Read the model definition and answer for the solid it produces. Units are mm, in the model's axes. Face numbers are marked on the shaded views. Round coordinates to 2 decimals unless told otherwise and drop trailing zeros. Order: outer loops, then holes, each group sorted by start corner. A loop starts at its lowest first (then second) coordinate and runs counter-clockwise, first axis right, second up. Notation, with made-up numbers: (46, 37) - (82, 37) arc R10 cw to (82, 44) - close; hole circle Ø2 at (32, 85.25). An arc over 180 degrees is marked (long way). Answer as a JSON object with one key per item and string values. Group by question number.
Q1. A cutting plane is placed at A-A on y = -93.5. Determine the outline of the cut face in (x, z), and give its area (3 significant figures).
Q2. A cutting plane is placed at C-C on x = -16. Determine the outline of the cut face in (y, z).
Q3. A cutting plane is placed at B-B on z = 5.5. Determine the outline of the cut face in (x, y).
Q4. Consider line 1 (Y direction, x = -47.5, z = 4.25); line 2 (X direction, y = -6, z = 6); line 3 (Z direction, x = -73, y = 64). Determine where each line is inside the solid, lowest interval first.
Q5. Given pin 1 Ø12 at (x, y) = (107, 92) entering from -Z; pin 2 Ø2.5 at (x, y) = (-133.08, 91.92) entering from -Z; pin 3 Ø10 at (x, y) = (70.5, 71.5) entering from +Z, each flat-ended and moving along its own axis, determine where each tip first touches the part or whether it passes through.
Q6. The mould has two halves that part along Y. Classify the marked faces 1 and 2: pulls with the +Y half, pulls with the -Y half, needs draft (parallel to the pull), parting line crosses it, or undercut.
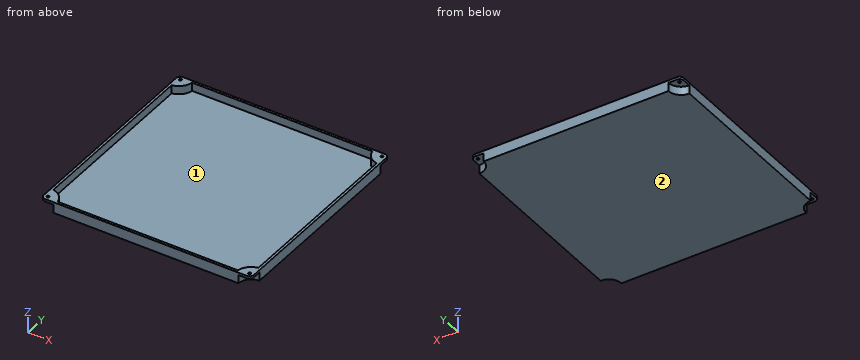
Autodesk Inventor part; units mm, degrees
ref_plane "YZ Plane" through (0, 0, 0) normal (1, 0, 0) x (0, 1, 0)
ref_plane "XZ Plane" through (0, 0, 0) normal (0, 1, 0) x (-1, 0, 0)
ref_plane "XY Plane" through (0, 0, 0) normal (0, 0, 1) x (1, 0, 0)
sketch "Sketch1" plane through (0, 0, 0) normal (0, 0, 1) x (1, 0, 0)
  line L0 (-123.0769, 96.9231) -> (96.9231, 96.9231)
  line L1 (111.9231, 81.9231) -> (111.9231, -138.0769)
  line L2 (96.9231, -153.0769) -> (-123.0769, -153.0769)
  line L3 (-138.0769, -138.0769) -> (-138.0769, 81.9231)
  arc A0 (-138.0769, 81.9231) -> (-123.0769, 96.9231) centre (-138.0769, 96.9231) ccw
  arc A1 (96.9231, 96.9231) -> (111.9231, 81.9231) centre (111.9231, 96.9231) ccw
  arc A2 (111.9231, -138.0769) -> (96.9231, -153.0769) centre (111.9231, -153.0769) ccw
  arc A3 (-123.0769, -153.0769) -> (-138.0769, -138.0769) centre (-138.0769, -153.0769) ccw
  point P0 (0, 0)
  dimension "d4" = 30
  dimension "d5" = 30
  dimension "d6" = 30
  dimension "d7" = 30
  dimension "d27" = 250
  dimension "d28" = 250
extrude "Extrusion1" add sketch "Sketch1" along normal blind 3
sketch "Sketch2" plane through (0, 0, 3) normal (0, 0, 1) x (1, 0, 0)
  line L0 (-123.0769, -153.0769) -> (96.9231, -153.0769)
  arc A0 (111.9231, -138.0769) -> (96.9231, -153.0769) centre (111.9231, -153.0769) ccw
  line L1 (111.9231, -138.0769) -> (111.9231, 81.9231)
  arc A1 (96.9231, 96.9231) -> (111.9231, 81.9231) centre (111.9231, 96.9231) ccw
  line L2 (96.9231, 96.9231) -> (-123.0769, 96.9231)
  arc A2 (-138.0769, 81.9231) -> (-123.0769, 96.9231) centre (-138.0769, 96.9231) ccw
  line L3 (-138.0769, 81.9231) -> (-138.0769, -138.0769)
  arc A3 (-123.0769, -153.0769) -> (-138.0769, -138.0769) centre (-138.0769, -153.0769) ccw
  line L4 (-120.3287, 93.9231) -> (94.1748, 93.9231)
  arc A4 (94.1748, 93.9231) -> (108.9231, 79.1748) centre (111.9231, 96.9231) ccw
  line L5 (108.9231, 79.1748) -> (108.9231, -135.3287)
  arc A5 (108.9231, -135.3287) -> (94.1748, -150.0769) centre (111.9231, -153.0769) ccw
  line L6 (94.1748, -150.0769) -> (-120.3287, -150.0769)
  arc A6 (-120.3287, -150.0769) -> (-135.0769, -135.3287) centre (-138.0769, -153.0769) ccw
  line L7 (-135.0769, -135.3287) -> (-135.0769, 79.1748)
  arc A7 (-135.0769, 79.1748) -> (-120.3287, 93.9231) centre (-138.0769, 96.9231) ccw
  point P0 (0, 0)
  dimension "d8" = 3
extrude "Extrusion2" add sketch "Sketch2" along normal blind 10
sketch "Sketch3" plane through (0, 0, 13) normal (0, 0, 1) x (1, 0, 0)
  line L0 (96.9231, 96.9231) -> (-123.0769, 96.9231)
  line L1 (-138.0769, 81.9231) -> (-138.0769, -138.0769)
  line L2 (111.9231, -138.0769) -> (111.9231, 81.9231)
  line L3 (-123.0769, -153.0769) -> (96.9231, -153.0769)
  arc A0 (111.9231, -138.0769) -> (96.9231, -153.0769) centre (111.9231, -153.0769) ccw
  arc A1 (-123.0769, -153.0769) -> (-138.0769, -138.0769) centre (-138.0769, -153.0769) ccw
  arc A2 (-138.0769, 81.9231) -> (-123.0769, 96.9231) centre (-138.0769, 96.9231) ccw
  arc A3 (96.9231, 96.9231) -> (111.9231, 81.9231) centre (111.9231, 96.9231) ccw
  line L4 (-138.0769, 96.9231) -> (111.9231, 96.9231)
  line L5 (111.9231, 96.9231) -> (111.9231, -153.0769)
  line L6 (111.9231, -153.0769) -> (-138.0769, -153.0769)
  line L7 (-138.0769, -153.0769) -> (-138.0769, 96.9231)
  point P0 (0, 0)
  point P1 (106.9231, 96.9231)
  point P2 (-133.0769, 86.9231)
  point P3 (116.9231, -143.0769)
  point P4 (111.9231, -138.0769)
  point P5 (-138.0769, -138.0769)
  point P6 (-123.0769, -153.0769)
  point P7 (-133.0769, 86.9231)
  point P8 (111.9231, 81.9231)
  point P9 (96.9231, 96.9231)
extrude "Extrusion3" add sketch "Sketch3" against normal blind 3 contours L4 L5 A3 | A2 L7 L4 | L5 L6 A0 | A1 L6 L7
fillet "Fillet1" radius 5 4 edges at (111.9231, -153.0769, 11.5) (-138.0769, -153.0769, 11.5) (111.9231, 96.9231, 11.5) (-138.0769, 96.9231, 11.5)
sketch "Sketch4" plane through (0, 0, 13) normal (0, 0, 1) x (1, 0, 0)
  arc A0 (-133.0769, 96.9231) -> (-138.0769, 91.9231) centre (-133.0769, 91.9231) ccw
  line L0 (-138.0769, 91.9231) -> (-138.0769, -148.0769)
  arc A1 (-138.0769, -148.0769) -> (-133.0769, -153.0769) centre (-133.0769, -148.0769) ccw
  line L1 (-133.0769, -153.0769) -> (106.9231, -153.0769)
  arc A2 (106.9231, -153.0769) -> (111.9231, -148.0769) centre (106.9231, -148.0769) ccw
  line L2 (111.9231, -148.0769) -> (111.9231, 91.9231)
  arc A3 (111.9231, 91.9231) -> (106.9231, 96.9231) centre (106.9231, 91.9231) ccw
  line L3 (106.9231, 96.9231) -> (-133.0769, 96.9231)
  line L4 (-120.3287, 93.9231) -> (94.1748, 93.9231)
  arc A4 (94.1748, 93.9231) -> (108.9231, 79.1748) centre (111.9231, 96.9231) ccw
  line L5 (108.9231, 79.1748) -> (108.9231, -135.3287)
  arc A5 (108.9231, -135.3287) -> (94.1748, -150.0769) centre (111.9231, -153.0769) ccw
  line L6 (94.1748, -150.0769) -> (-120.3287, -150.0769)
  arc A6 (-120.3287, -150.0769) -> (-135.0769, -135.3287) centre (-138.0769, -153.0769) ccw
  line L7 (-135.0769, -135.3287) -> (-135.0769, 79.1748)
  arc A7 (-135.0769, 79.1748) -> (-120.3287, 93.9231) centre (-138.0769, 96.9231) ccw
  circle A8 centre (-133.0769, 91.9231) radius 1.6
  circle A9 centre (-133.0769, -148.0769) radius 1.6
  circle A10 centre (106.9231, 91.9231) radius 1.6
  circle A11 centre (106.9231, -148.0769) radius 1.6
  point P0 (0, 0)
  dimension "d14" = 3.2
  dimension "d15" = 5
  dimension "d16" = 5
  dimension "d19" = 240
  dimension "d22" = 240
extrude "Extrusion4" cut sketch "Sketch4" against normal blind 3 contours A8 | A9 | A10 | A11
properties part number "Enclosure cover"
Result set:
{
 "1": {"outline": "(-138.08, 0) - (111.92, 0) - (111.92, 13) - (108.92, 13) - (108.92, 3) - (-135.08, 3) - (-135.08, 13) - (-138.08, 13) - close", "area": "810 mm²"},
 "2": {"outline": "(-153.08, 0) - (96.92, 0) - (96.92, 13) - (93.92, 13) - (93.92, 3) - (-150.08, 3) - (-150.08, 13) - (-153.08, 13) - close"},
 "3": {"outline": "(-138.08, -138.08) arc R15 cw to (-123.08, -153.08) - (96.92, -153.08) arc R15 cw to (111.92, -138.08) - (111.92, 81.92) arc R15 cw to (96.92, 96.92) - (-123.08, 96.92) arc R15 cw to (-138.08, 81.92) - close; hole (-135.08, -135.33) arc R18 cw to (-120.33, -150.08) - (94.17, -150.08) arc R18 cw to (108.92, -135.33) - (108.92, 79.17) arc R18 cw to (94.17, 93.92) - (-120.33, 93.92) arc R18 cw to (-135.08, 79.17) - close"},
 "4": {"line 1": "y = -153.08 to -150.08, 93.92 to 96.92", "line 2": "x = -138.08 to -135.08, 108.92 to 111.92", "line 3": "z = 0 to 3"},
 "5": {"pin 1": "stops at z = 10", "pin 2": "passes through", "pin 3": "stops at z = 3"},
 "6": {"face 1": "undercut", "face 2": "needs draft"}
}
